The model under review builds one solid part; all positions refer to its coordinate system, in mm. Face numbers are marked on the shaded views. A direction names the side the tool comes from. Coordinates: 2 decimals unless noted, no trailing zeros. Loops run counter-clockwise (first coordinate to the right, second up) from the corner with the lowest first, then second, coordinate; pieces in that order, holes last. Notation, with made-up numbers: (57.25, 59) - (95.25, 59) arc R16 cw to (95.25, 88) - close; hole circle Ø7 at (-28, -4). An arc over 180 degrees is marked (long way). One line per item, written item: value. Start each with the question number.
1. We need section B-B, the plane z = 1. Give the boundary of the cut face in (x, y).
2. We need section A-A, the plane y = 27.5. Give the boundary of the cut face in (x, z), then the cut area to 3 significant figures.
3. We need section D-D, the plane x = 6.5. Give the boundary of the cut face in (y, z), then the cut area to 4 significant figures.
4. We need section C-C, the plane y = 37.5. Count the separate pieces of the cut face and the enclosed holes in it, then the cut area to 3 significant figures.
5. For the marked faces 1, 2 and 3, list the 3-axis set-ups (+Z, -Z, +X, -X, +Y, -Y) from which the entire face can be reached by the end or side of a thin tool; tool diameter is ignored.
6. To check wall thickness, follow line 1 (X direction, y = 47, z = 14); line 2 (X direction, y = 32.5, z = 2.5); line 3 (Z direction, x = 29.5, y = 31.5). State the ranges of each line that lie inside material, in increasing order.
7. Mouldability with a two-part tool opening along X and no side actions: class the marked faces 4, 5 and 6 as +X half, -X half, draft (parallel to the pull), parting line (faces both ways), or undercut.
8. Insertion check: P1, Ø1.8, axis at x = -56.5, z = 13.5, coming from the +Y side; P2, Ø6, axis at x = 16, z = -8, coming from the +Y side. Each pin has a flat end and moves straight along its axis. Give the tip position at first contact, or say it passes through.
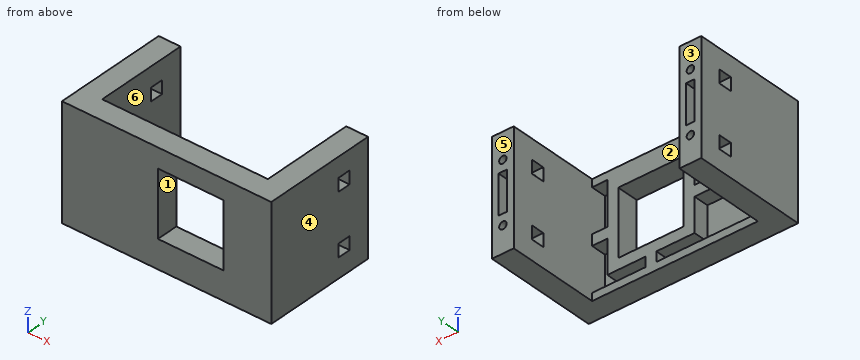
from build123d import *

# Parameters (mm, degrees)
SKETCH1_W           = 96
SKETCH1_H           = 52
BOSS_EXTRUDE1_DEPTH = 10
SKETCH3_W           = 30
SKETCH3_H           = 30
CUT_EXTRUDE1_DEPTH  = 10
SKETCH4_W           = 10
SKETCH4_H           = 52
BOSS_EXTRUDE2_DEPTH = 42.5
CUT_EXTRUDE2_DEPTH  = 25
SKETCH10_W          = 6
SKETCH10_H          = 6
CUT_EXTRUDE7_DEPTH  = 113.464438824
SKETCH11_R          = 1.7
SKETCH11_W          = 4
SKETCH11_H          = 18
CUT_EXTRUDE8_DEPTH  = 60
SKETCH14_W          = 96
SKETCH14_H          = 52
SKETCH14_W_2        = 30
SKETCH14_H_2        = 30
BOSS_EXTRUDE3_DEPTH = 3


with BuildPart() as part:
    # Sketch1 → Boss-Extrude1 (new body)
    with BuildSketch(Plane(origin=(0, 0, 0), x_dir=(1, 0, 0), z_dir=(0, 1, 0))):
        with Locations((-13, 0)):
            Rectangle(SKETCH1_W, SKETCH1_H)
    extrude(amount=BOSS_EXTRUDE1_DEPTH)

    # Sketch3 → Cut-Extrude1 (cut)
    with BuildSketch(Plane(origin=(0, 10, 0), x_dir=(1, 0, 0), z_dir=(0, 1, 0))):
        with Locations((-2, -2)):
            Rectangle(SKETCH3_W, SKETCH3_H)
    extrude(amount=-CUT_EXTRUDE1_DEPTH, mode=Mode.SUBTRACT)

    # Sketch4 → Boss-Extrude2 (add)
    with BuildSketch(Plane(origin=(0, 10, 0), x_dir=(1, 0, 0), z_dir=(0, 1, 0))):
        with Locations((30, 0)):
            Rectangle(SKETCH4_W, SKETCH4_H)
        with Locations((-56, 0)):
            Rectangle(SKETCH4_W, SKETCH4_H)
    extrude(amount=BOSS_EXTRUDE2_DEPTH)

    # Sketch5 → Cut-Extrude2 (cut)
    with BuildSketch(Plane(origin=(0, 10, 0), x_dir=(1, 0, 0), z_dir=(0, 1, 0))):
        Polygon((25, 22.5), (0.5, 22.5), (0.5, 18), (18, 18), (18, 2.5), (25, 2.5), align=None)
        Polygon((-4.5, 22.5), (-51, 22.5), (-51, 2.5), (-22, 2.5), (-22, 18), (-4.5, 18), align=None)
        Polygon((-22, -2.5), (-51, -2.5), (-51, -22.5), (-22, -22.5), (-22, -20), align=None)
        Polygon((25, -22.5), (25, -2.5), (18, -2.5), (18, -20), (18, -22.5), align=None)
    extrude(amount=-CUT_EXTRUDE2_DEPTH, mode=Mode.SUBTRACT)

    # Sketch10 → Cut-Extrude7 (cut, through all)
    with BuildSketch(Plane(origin=(35, 0, 0), x_dir=(0, 0, -1), z_dir=(1, 0, 0))):
        with Locations((14, 39.5)):
            Rectangle(SKETCH10_W, SKETCH10_H)
        with Locations((-14, 39.5)):
            Rectangle(SKETCH10_W, SKETCH10_H)
    extrude(amount=-CUT_EXTRUDE7_DEPTH, mode=Mode.SUBTRACT)

    # Sketch11 → Cut-Extrude8 (cut)
    with BuildSketch(Plane(origin=(0, 52.5, 0), x_dir=(1, 0, 0), z_dir=(0, 1, 0))):
        with Locations(Location((-56, 14, 0), (0, 0, 270))):
            Circle(SKETCH11_R)
        with Locations(Location((-56, -14, 0), (0, 0, 270))):
            Circle(SKETCH11_R)
        with Locations(Location((30, -14, 0), (0, 0, 270))):
            Circle(SKETCH11_R)
        with Locations(Location((30, 14, 0), (0, 0, 270))):
            Circle(SKETCH11_R)
        with Locations((-56, 0)):
            Rectangle(SKETCH11_W, SKETCH11_H)
        with Locations((30, 0)):
            Rectangle(SKETCH11_W, SKETCH11_H)
    extrude(amount=-CUT_EXTRUDE8_DEPTH, mode=Mode.SUBTRACT)

    # Sketch14 → Boss-Extrude3 (add)
    with BuildSketch(Plane.XZ):
        with Locations((-13, 0)):
            Rectangle(SKETCH14_W, SKETCH14_H)
        with Locations((-2, 2)):
            Rectangle(SKETCH14_W_2, SKETCH14_H_2, mode=Mode.SUBTRACT)
    extrude(amount=-BOSS_EXTRUDE3_DEPTH)


solid = part.part
Findings below:
1. outline: (-61, 0) - (-17, 0) - (-17, 10) - (-51, 10) - (-51, 52.5) - (-54, 52.5) - (-54, 3) - (-58, 3) - (-58, 52.5) - (-61, 52.5) - close; (13, 0) - (35, 0) - (35, 52.5) - (32, 52.5) - (32, 3) - (28, 3) - (28, 52.5) - (25, 52.5) - (25, 10) - (13, 10) - close
2. outline: (-61, -26) - (-51, -26) - (-51, 26) - (-61, 26) - close; (25, -26) - (35, -26) - (35, 26) - (25, 26) - close; hole (-58, -9) - (-54, -9) - (-54, 9) - (-58, 9) - close; hole circle Ø3.4 at (-56, -14); hole circle Ø3.4 at (-56, 14); hole (28, -9) - (32, -9) - (32, 9) - (28, 9) - close; hole circle Ø3.4 at (30, -14); hole circle Ø3.4 at (30, 14)
2. area: 860 mm2
3. outline: (0, -26) - (10, -26) - (10, -22.5) - (3, -22.5) - (3, -18) - (10, -18) - (10, -13) - (0, -13) - close; (0, 17) - (10, 17) - (10, 26) - (0, 26) - close
3. area: 188.5 mm2
4. separate pieces: 6
4. enclosed holes: 2
4. area: 656 mm2
5. face 1: +Y, -Y
5. face 2: +Z, -Z, +Y
5. face 3: +Z, -Z, +X, -X, +Y
6. line 1: -61 to -57.7, -54.3 to -51, 25 to 28.3, 31.7 to 35
6. line 2: -61 to -58, -54 to -51, 25 to 28, 32 to 35
6. line 3: -26 to -15.62, -12.38 to -9, 9 to 12.38, 15.62 to 26
7. face 4: +X half
7. face 5: draft
7. face 6: undercut
8. P1: y = 3
8. P2: y = 10
